Autodesk Inventor part; units mm, degrees
ref_plane "YZ Plane" through (0, 0, 0) normal (1, 0, 0) x (0, 1, 0)
ref_plane "XZ Plane" through (0, 0, 0) normal (0, 1, 0) x (-1, 0, 0)
ref_plane "XY Plane" through (0, 0, 0) normal (0, 0, 1) x (1, 0, 0)
sketch "Szkic1" plane through (0, 0, 0) normal (0, 1, 0) x (-1, 0, 0)
  circle A0 centre (0, 0) radius 35.5
  line L0 (0, 18.75) -> (0, -18.75) construction
  line L1 (-28, 0) -> (28, 0) construction
  line L2 (-28, -18.75) -> (28, -18.75)
  line L3 (-28, 18.75) -> (-28, -18.75)
  line L4 (28, 18.75) -> (28, -18.75)
  line L5 (0, 18.75) -> (28, 18.75)
  line L6 (0, 18.75) -> (-28, 18.75)
  line L7 (0, 18.75) -> (0, 28.75) construction
  line L8 (17, 28.75) -> (-17, 28.75)
  line L9 (17, 28.75) -> (17, 18.75)
  line L10 (-17, 28.75) -> (-17, 18.75)
  line L11 (0, -18.75) -> (0, -28.75) construction
  line L12 (-17, -28.75) -> (17, -28.75)
  line L13 (17, -28.75) -> (17, -18.75)
  line L14 (-17, -28.75) -> (-17, -18.75)
  point P0 (0, 0)
  dimension "d0" = 71
  dimension "d1" = 37.5
  dimension "d2" = 56
  dimension "d3" = 10
  dimension "d4" = 34
  dimension "d5" = 10
  dimension "d6" = 34
extrude "Wyciągnięcie proste1" add sketch "Szkic1" along normal blind 10
extrude "Wyciągnięcie proste2" add sketch "Szkic1" against normal blind 3 contours A0 | L3 L6 L5 L4 L2
sketch "Szkic2" plane through (0, 10, 0) normal (0, 1, 0) x (1, 0, 0)
  line L0 (32, 0) -> (-32, 0) construction
  circle A0 centre (0, 0) radius 35.5
  line L1 (-32, -10) -> (-32, 10)
  line L2 (32, -10) -> (32, 10)
  line L3 (32, -10) -> (34.0624, -10)
  line L4 (32, 10) -> (34.0624, 10)
  line L5 (-32, -10) -> (-34.0624, -10)
  line L6 (-32, 10) -> (-34.0624, 10)
  point P0 (0, 0)
  dimension "d11" = 64
  dimension "d12" = 71
  dimension "d13" = 20
  dimension "d14" = 20
extrude "Wyciągnięcie proste3" add sketch "Szkic2" along normal blind 10 contours A0 L3 L2 L4 | L6 L1 L5 A0
sketch "Szkic3" plane through (-32, 10, 10) normal (1, 0, 0) x (0, 0, -1)
  line L0 (0, 0) -> (10, 0) construction
  line L1 (10, 0) -> (10, 5) construction
  circle A0 centre (10, 5) radius 1
  point P0 (10, -10)
  dimension "d17" = 10
  dimension "d18" = 5
  dimension "d19" = 0
  dimension "d20" = 10
  dimension "d21" = 2
extrude "Wyciągnięcie proste4" cut sketch "Szkic3" along normal through all both and the other way through all
properties part number "007-002"
Geometry: final body of the model. Coordinates: model frame, mm. A direction names the side the tool comes from. Round coordinates to 2 decimals unless told otherwise and drop trailing zeros. Write each loop counter-clockwise with the first axis right and the second up, starting at its lowest first coordinate (ties: lowest second). Pieces come first, ordered by that corner, then holes. Notation, with made-up numbers: M 27,-12.5 L 41,-12.5 A18 ccw 41,-0.5 Z; hole C -32.5,39.5 d4. An arc over 180 degrees is marked long. Answer in a Markdown table with one row per item. Add a question column.
(1) Reachability of faces 4 (the face through (-33, 15, -10)), 5 (the face through (32, 13.8, 0.1)), 6 (the face through (-28, 5, 0)), 7 (the face through (-17, 4, 24)), 8 (the face through (33, 15, 10)) from +Z, -Z, +X, -X, +Y, -Y: full face, straight path, thin tool, end or side. Return the list, or none.
(2) Ray query, L1, parallel to Y at x = 32.7, z = 0; L2, parallel to Z at x = -34, y = 15; L3, parallel to Y at x = -2, z = -12.5. Return the intervals inside material, ascending.
(3) Contact query for flat-ended pins moving along their axis: pin 1 (5 mm diameter, centred on y = 3, z = 6.5, fed in from -X); pin 2 (5 mm diameter, centred on y = 7.5, z = -3, fed in from +X); pin 3 (11 mm diameter, centred on x = 24.5, y = 5, fed in from -Z). Output: stop coordinate, or through.
(4) Cut plane B-B, the plane y = 7.25. Return the cut outline in (x, z), then the cut area to 3 significant figures.
(5) Cut plane D-D, the plane z = 0. Return the cut outline in (x, y), then the cut area to 3 significant figures.
(6) Draft query along Z for faces 1 (the face through (-33, 15, 10)), 2 (the face through (33, 15, -10)), 3 (the face through (0, 4, -28.75)). Return one class per face: pulls with the +Z half, pulls with the -Z half, needs draft (parallel to the pull), parting line crosses it, or undercut.
(7) Cut plane A-A, the plane x = 0. Return the cut outline in (y, z), then the cut area to 3 significant figures.
(8) Cut plane C-C, the plane z = 20. Return the cut outline in (x, y).
Established:
| question | item | result |
|---|---|---|
| 1 | face 4 | -Z, +X, -X, +Y |
| 1 | face 5 | +Z, -Z, +Y |
| 1 | face 6 | +Y |
| 1 | face 7 | +Y, -Y |
| 1 | face 8 | +Z, +X, -X, +Y |
| 2 | L1 | -3 to 14, 16 to 20 |
| 2 | L2 | -10 to -1, 1 to 10 |
| 2 | L3 | -3 to 0 |
| 3 | pin 1 | x = -35.27 |
| 3 | pin 2 | x = 35.5 |
| 3 | pin 3 | z = -29.99 |
| 4 | outline | C 0,0 d71; hole M -28,-18.75 L -17,-18.75 L -17,-28.75 L 17,-28.75 L 17,-18.75 L 28,-18.75 L 28,18.75 L 17,18.75 L 17,28.75 L -17,28.75 L -17,18.75 L -28,18.75 Z |
| 4 | area | 1,180 mm² |
| 5 | outline | M -35.5,-3 L 35.5,-3 L 35.5,14 L 32,14 L 32,10 L 28,10 L 28,0 L -28,0 L -28,10 L -32,10 L -32,14 L -35.5,14 Z; M -35.5,16 L -32,16 L -32,20 L -35.5,20 Z; M 32,16 L 35.5,16 L 35.5,20 L 32,20 Z |
| 5 | area | 419 mm² |
| 6 | face 1 | pulls with the +Z half |
| 6 | face 2 | pulls with the -Z half |
| 6 | face 3 | undercut |
| 7 | outline | M -3,-35.5 L 10,-35.5 L 10,-28.75 L -3,-28.75 Z; M -3,-18.75 L 0,-18.75 L 0,18.75 L -3,18.75 Z; M -3,28.75 L 10,28.75 L 10,35.5 L -3,35.5 Z |
| 7 | area | 288 mm² |
| 8 | outline | M -29.33,-3 L -17,-3 L -17,10 L -29.33,10 Z; M 17,-3 L 29.33,-3 L 29.33,10 L 17,10 Z |
